Part model, mm, in its own coordinate system. Coordinates: 2 decimals unless noted, no trailing zeros. Loops run counter-clockwise (first coordinate to the right, second up) from the corner with the lowest first, then second, coordinate; pieces in that order, holes last. Notation, with made-up numbers: M 30.5,11.25 L 76.5,11.25 A14 cw 76.5,20.25 Z; hole C 61,29.25 d4. An arc over 180 degrees is marked long. Answer as CSV lines item,"result". Start each with the question number.
from build123d import *

# Parameters (mm, degrees)
SKETCH1_W                            = 143.4
SKETCH1_H                            = 102.4
SKETCH1_W_2                          = 124
SKETCH1_H_2                          = 81.7
BOSS_EXTRUDE1_DEPTH                  = 13
SKETCH2_W                            = 128.4
SKETCH2_H                            = 86.1
CUT_EXTRUDE1_DEPTH                   = 12.5
SKETCH3_W                            = 143.4
SKETCH3_H                            = 102.4
SKETCH3_W_2                          = 130.1
SKETCH3_H_2                          = 87.7
CUT_EXTRUDE3_DEPTH                   = 8.3
FILLET1_R                            = 1
FILLET2_R                            = 1.5
FILLET3_R                            = 3
SKETCH4_W                            = 60
SKETCH4_H                            = 8.15
CUT_EXTRUDE4_DEPTH                   = 3.7
CHAMFER1_SIZE                        = 6.4
CHAMFER1_SIZE2                       = 3.695041723
CHAMFER2_SIZE                        = 6.4
CHAMFER2_SIZE2                       = 3.695041723
SKETCH5_R                            = 1.5
CUT_EXTRUDE5_DEPTH                   = 0.5
CHAMFER3_SIZE                        = 2
F_3_7_3_7_DIAMETER_HOLE1_D           = 3.7
F_3_7_3_7_DIAMETER_HOLE1_DEPTH       = 3
F_3_7_3_7_DIAMETER_HOLE1_CSINK_D     = 3.75
F_3_7_3_7_DIAMETER_HOLE1_CSINK_ANGLE = 90
F_3_7_3_7_DIAMETER_HOLE1_TIP         = 1.111592145


with BuildPart() as part:
    # Sketch1 → Boss-Extrude1 (new body)
    with BuildSketch(Plane(origin=(0, 0, 0), x_dir=(1, 0, 0), z_dir=(0, 1, 0))):
        Rectangle(SKETCH1_W, SKETCH1_H)
        Rectangle(SKETCH1_W_2, SKETCH1_H_2, mode=Mode.SUBTRACT)
    extrude(amount=BOSS_EXTRUDE1_DEPTH)

    # Sketch2 → Cut-Extrude1 (cut)
    with BuildSketch(Plane(origin=(0, 13, 0), x_dir=(1, 0, 0), z_dir=(0, 1, 0))):
        Rectangle(SKETCH2_W, SKETCH2_H)
    extrude(amount=-CUT_EXTRUDE1_DEPTH, mode=Mode.SUBTRACT)

    # Sketch3 → Cut-Extrude3 (cut)
    with BuildSketch(Plane.XZ):
        Rectangle(SKETCH3_W, SKETCH3_H)
        Rectangle(SKETCH3_W_2, SKETCH3_H_2, mode=Mode.SUBTRACT)
    extrude(amount=-CUT_EXTRUDE3_DEPTH, mode=Mode.SUBTRACT)

    # Fillet1
    fillet1_edges = [part.edges().sort_by_distance(p)[0] for p in [
        (-62, 0.25, 40.85),
        (62, 0.25, 40.85),
        (-62, 0.25, -40.85),
        (62, 0.25, -40.85),
    ]]
    fillet(fillet1_edges, radius=FILLET1_R)

    # Fillet2
    fillet2_edges = [part.edges().sort_by_distance(p)[0] for p in [
        (64.2, 6.75, -43.05),
        (64.2, 6.75, 43.05),
        (-64.2, 6.75, 43.05),
        (-64.2, 6.75, -43.05),
    ]]
    fillet(fillet2_edges, radius=FILLET2_R)

    # Fillet3
    fillet3_edges = [part.edges().sort_by_distance(p)[0] for p in [
        (65.05, 4.15, -43.85),
        (-65.05, 4.15, -43.85),
        (-65.05, 4.15, 43.85),
        (65.05, 4.15, 43.85),
        (71.7, 10.65, 51.2),
        (-71.7, 10.65, 51.2),
        (-71.7, 10.65, -51.2),
        (71.7, 10.65, -51.2),
    ]]
    fillet(fillet3_edges, radius=FILLET3_R)

    # Sketch4 → Cut-Extrude4 (cut)
    with BuildSketch(Plane(origin=(0, 13, 0), x_dir=(1, 0, 0), z_dir=(0, 1, 0))):
        with Locations((0, 47.125)):
            Rectangle(SKETCH4_W, SKETCH4_H)
    cut_extrude4 = extrude(amount=-CUT_EXTRUDE4_DEPTH, mode=Mode.SUBTRACT)

    # Mirror1: Cut-Extrude4 across plane
    add(cut_extrude4.mirror(Plane.XY), mode=Mode.SUBTRACT)

    # Chamfer1
    chamfer1_edges = [part.edges().sort_by_distance(p)[0] for p in [
        (-30, 9.3, -47.125),
        (30, 9.3, -47.125),
    ]]
    chamfer1_side = [part.faces().sort_by_distance(p)[0] for p in [
        (0, 9.3, -47.125),
    ]]
    chamfer(chamfer1_edges, length=CHAMFER1_SIZE, length2=CHAMFER1_SIZE2, reference=chamfer1_side[0])

    # Chamfer2
    chamfer2_edges = [part.edges().sort_by_distance(p)[0] for p in [
        (30, 9.3, 47.125),
        (-30, 9.3, 47.125),
    ]]
    chamfer2_side = [part.faces().sort_by_distance(p)[0] for p in [
        (0, 9.3, 47.125),
    ]]
    chamfer(chamfer2_edges, length=CHAMFER2_SIZE, length2=CHAMFER2_SIZE2, reference=chamfer2_side[0])

    # Sketch5 → Cut-Extrude5 (cut)
    with BuildSketch(Plane(origin=(0, 13, 0), x_dir=(1, 0, 0), z_dir=(0, 1, 0))):
        with Locations(Location((69.2, -16.7, 0), (0, 0, 270))):
            Circle(SKETCH5_R)
    extrude(amount=-CUT_EXTRUDE5_DEPTH, mode=Mode.SUBTRACT)

    # Chamfer3
    chamfer3_edges = [part.edges().sort_by_distance(p)[0] for p in [
        (46.35, 13, 43.05),
        (63.760660172, 13, 42.610660172),
        (64.2, 13, 0),
        (63.760660172, 13, -42.610660172),
        (46.35, 13, -43.05),
        (-46.35, 13, -43.05),
        (-46.35, 13, 43.05),
        (-63.760660172, 13, -42.610660172),
        (-63.760660172, 13, 42.610660172),
        (-64.2, 13, 0),
    ]]
    chamfer(chamfer3_edges, length=CHAMFER3_SIZE)

    # Ø3.7 (3.7) Diameter Hole1
    with Locations(Plane(origin=(0, 8.3, 0), x_dir=(-1, 0, 0), z_dir=(0, -1, 0))):
        with Locations((-68, 47.5), (-68, -47.5), (68, 47.5), (68, -47.5)):
            CounterSinkHole(F_3_7_3_7_DIAMETER_HOLE1_D / 2, F_3_7_3_7_DIAMETER_HOLE1_CSINK_D / 2, depth=F_3_7_3_7_DIAMETER_HOLE1_DEPTH, counter_sink_angle=F_3_7_3_7_DIAMETER_HOLE1_CSINK_ANGLE)
            with Locations((0, 0, -(F_3_7_3_7_DIAMETER_HOLE1_DEPTH + F_3_7_3_7_DIAMETER_HOLE1_TIP / 2))):  # 118° drill point
                Cone(0, F_3_7_3_7_DIAMETER_HOLE1_D / 2, F_3_7_3_7_DIAMETER_HOLE1_TIP, mode=Mode.SUBTRACT)


solid = part.part
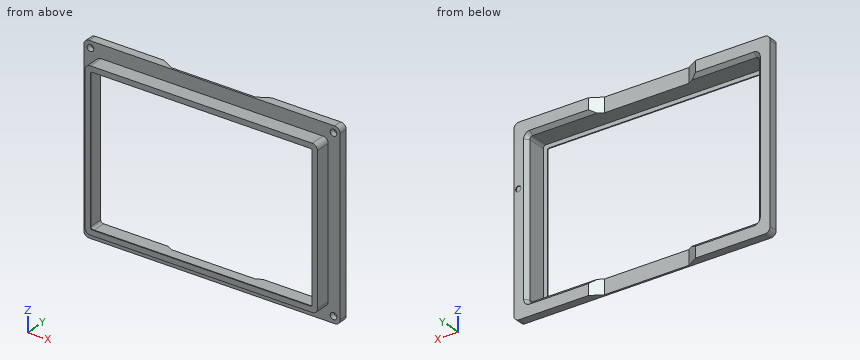
Q1. Wall check: L1, parallel to X at y = 9.05, z = -47.5; L2, parallel to Z at x = 68, y = 10.5; L3, parallel to Z at x = 54, y = 9.25. Give the ranges that are in metal, low to high.
Q2. Slice it at A-A, the plane x = -1. Write the cut outline in (y, z), and give its area (3 significant figures).
Q3. Slice it at B-B, the plane z = 16.7. Write the cut outline in (x, y), and give its area (3 significant figures).
Q4. Slice it at D-D, the plane z = -33. Write the cut outline in (x, y), and give its area (3 significant figures).
Q5. Slice it at C-C, the plane y = 2.25. Write the cut outline in (x, z).
Q6. Flat gauge pins, fed straight in: P1, Ø5, axis at x = -23, y = 4.5, coming from the -Z side; P2, Ø6.5, axis at x = -5.5, z = -45, coming from the +Y side; P3, Ø3.5, axis at x = -68, z = 47.5, coming from the -Y side. Where does each tip first touch, or does it go through?
Solved:
1,L1,"x = -71.7 to -69.85, -66.15 to 66.15, 69.85 to 71.7"
1,L2,"z = -51.2 to -49.35, -45.65 to 45.65, 49.35 to 51.2"
1,L3,"z = -51.2 to -43.05, 43.05 to 51.2"
2,outline,"M 0,-43.85 L 8.3,-43.85 L 8.3,-51.2 L 9.3,-51.2 L 9.3,-43.05 L 0.5,-43.05 L 0.5,-40.85 L 0,-40.85 Z; M 0,40.85 L 0.5,40.85 L 0.5,43.05 L 9.3,43.05 L 9.3,51.2 L 8.3,51.2 L 8.3,43.85 L 0,43.85 Z"
2,area,"31.8 mm2"
3,outline,"M -71.7,8.3 L -65.05,8.3 L -65.05,0 L -62,0 L -62,0.5 L -64.2,0.5 L -64.2,11 L -66.2,13 L -71.7,13 Z; M 62,0 L 65.05,0 L 65.05,8.3 L 71.7,8.3 L 71.7,13 L 70.7,13 L 70.7,12.5 L 67.7,12.5 L 67.7,13 L 66.2,13 L 64.2,11 L 64.2,0.5 L 62,0.5 Z"
3,area,"81.3 mm2"
4,outline,"M -71.7,8.3 L -65.05,8.3 L -65.05,0 L -62,0 L -62,0.5 L -64.2,0.5 L -64.2,11 L -66.2,13 L -71.7,13 Z; M 62,0 L 65.05,0 L 65.05,8.3 L 71.7,8.3 L 71.7,13 L 66.2,13 L 64.2,11 L 64.2,0.5 L 62,0.5 Z"
4,area,"82.8 mm2"
5,outline,"M -65.05,-40.85 A3 ccw -62.05,-43.85 L 62.05,-43.85 A3 ccw 65.05,-40.85 L 65.05,40.85 A3 ccw 62.05,43.85 L -62.05,43.85 A3 ccw -65.05,40.85 Z; hole M -64.2,-41.55 A1.5 ccw -62.7,-43.05 L 62.7,-43.05 A1.5 ccw 64.2,-41.55 L 64.2,41.55 A1.5 ccw 62.7,43.05 L -62.7,43.05 A1.5 ccw -64.2,41.55 Z"
6,P1,"stops at z = -43.85"
6,P2,"stops at y = 9.3"
6,P3,"stops at y = 11.36"
